CAD build for the part. Positions are in the model's coordinates, mm. A direction names the side the tool comes from. Give positions to 0.01 mm unless a question says otherwise; leave off trailing zeros. Write each loop counter-clockwise with the first axis right and the second up, starting at its lowest first coordinate (ties: lowest second). Pieces come first, ordered by that corner, then holes. Notation, with made-up numbers: (57.5, -25) - (116.5, -25) arc R32 ccw to (116.5, 7) - close; hole circle Ø8 at (74.25, -6). An arc over 180 degrees is marked (long way). Put each result on its own line as item: value. Start each with the question number.
1. Wall check: line 1 (X direction, y = 60, z = 14); line 2 (X direction, y = 100, z = 3); line 3 (Z direction, x = 29, y = 66). Give the ranges that are in metal, low to high.
2. Drop flat-ended pins along their axis: pin 1 (6 mm diameter, centred on y = 28, z = 25.5, fed in from -X); pin 2 (3 mm diameter, centred on x = 20, z = 17, fed in from +Y); pin 3 (12 mm diameter, centred on x = -5, z = 45, fed in from +Y); pin 4 (17 mm diameter, centred on x = 19.5, y = 98, fed in from +Z). Give the stop position or say it passes through.
3. Cut at B-B on y = 60. List the corners of the cut face in (x, z), and give its area (3 significant figures).
4. Tool access for faces 5 (the cylindrical face through (38, 60.8, 2.1)), 6 (the flat face through (-0.6, 15, 27.8)): list every direction of +Z, -Z, +X, -X, +Y, -Y with a clear straight run to the whole face (end or side of a thin tool).
5. Mould opens along X. For faces 1 (the flat face through (31.01, 7.4, 35.92)), 2 (the flat face through (-30.76, 7.4, 36.37)), 3 (the cylindrical face through (10.651, 104.868, 3.944)), 4 (the flat face through (-1, 80, 17)) say: +X half, -X half, draft (parallel to the pull), parting line (faces both ways), or undercut.
6. Cut at A-A on x = 17.5. List the corners of the cut face in (y, z).
7. Cut at D-D on x = -2.5. List the corners of the cut face in (y, z), and give its area (3 significant figures).
8. Cut at C-C on z = 31. List the corners of the cut face in (x, y).
from build123d import *

# Parameters (mm, degrees)
F0_W           = 80
F0_H           = 20
F1_DEPTH       = 120
F0_R           = 12
F2_DEPTH       = 15
F3_W           = 80
F3_H           = 40
F4_DEPTH       = 12
F5_R           = 6
F6_R           = 7
F7_R           = 8
F8_DEPTH       = 20
F10_R          = 20
F11_DEPTH      = 108.7579344444
F11_DEPTH_BACK = 27.4711870131


with BuildPart() as f1:
    # F0 (on Front) → F1 (new body)
    with BuildSketch(Plane.XZ):
        with Locations((0, 10)):
            Rectangle(F0_W, F0_H)
    extrude(amount=-F1_DEPTH)

    # F0 (on Front) → F2 (join)
    with BuildSketch(Plane.XZ):
        with BuildLine():
            Line((40, 20), (21.7702481089, 52.2904962177))
            ThreePointArc((21.7702481089, 52.2904962177), (0, 65), (-21.7702481089, 52.2904962177))
            Line((-21.7702481089, 52.2904962177), (-40, 20))
            Line((-40, 20), (40, 20))
        make_face()
        with Locations((0, 40)):
            Circle(F0_R, mode=Mode.SUBTRACT)
    extrude(amount=-F2_DEPTH)

    # F3 (on face) → F4 (cut)
    with BuildSketch(Plane.XY.offset(20)):
        with Locations((0, 100)):
            Rectangle(F3_W, F3_H)
    extrude(amount=-F4_DEPTH, mode=Mode.SUBTRACT)

    # F5
    f5_edges = [f1.edges().sort_by_distance(p)[0] for p in [
        (0, 80, 8),
    ]]
    fillet(f5_edges, radius=F5_R)

    # F6
    f6_edges = [f1.edges().sort_by_distance(p)[0] for p in [
        (40, 60, 0),
        (-40, 60, 0),
    ]]
    fillet(f6_edges, radius=F6_R)

    # F7 (on face) → F8 (cut, through all)
    with BuildSketch(Plane(origin=(0, 0, 0), x_dir=(1, 0, 0), z_dir=(0, 0, -1))):
        with Locations((17, -60)):
            Circle(F7_R)
        with Locations((17, -100)):
            Circle(F7_R)
        with Locations((-17, -100)):
            Circle(F7_R)
        with Locations((-17, -60)):
            Circle(F7_R)
    extrude(amount=-F8_DEPTH, mode=Mode.SUBTRACT)

    # F10 (on line) → F11 (cut, two sides)
    with BuildSketch(Plane(origin=(0, 0, 0), x_dir=(1, 0, 0), z_dir=(0, -0.906307787, 0.4226182617))) as f11_sk:
        Circle(F10_R)
    extrude(amount=-F11_DEPTH, mode=Mode.SUBTRACT)
    extrude(f11_sk.sketch, amount=F11_DEPTH_BACK, mode=Mode.SUBTRACT)


solid = f1.part
Report:
1. line 1: x = -40 to -25, -9 to 9, 25 to 40
1. line 2: x = -38.74 to -25, -9 to 9, 25 to 38.74
1. line 3: z = 0 to 20
2. pin 1: passes through
2. pin 2: stops at y = 80
2. pin 3: stops at y = 15
2. pin 4: stops at z = 8
3. outline: (-40, 7) arc R7 ccw to (-33, 0) - (-25, 0) - (-25, 20) - (-40, 20) - close; (-9, 0) - (9, 0) - (9, 20) - (-9, 20) - close; (25, 0) - (33, 0) arc R7 ccw to (40, 7) - (40, 20) - (25, 20) - close
3. area: 939 mm²
4. face 5: -Z, +X, +Y, -Y
4. face 6: +Z, +X, -X, +Y
5. face 1: +X half
5. face 2: -X half
5. face 3: undercut
5. face 4: draft
6. outline: (0, 10.68) - (22.91, 0) - (52.02, 0) - (52.02, 20) - (15, 20) - (15, 57.85) - (0, 57.85) - close; (67.98, 0) - (92.02, 0) - (92.02, 8) - (86, 8) arc R6 cw to (80, 14) - (80, 20) - (67.98, 20) - close; (107.98, 0) - (120, 0) - (120, 8) - (107.98, 8) - close
7. outline: (0, 21.89) - (46.95, 0) - (120, 0) - (120, 8) - (86, 8) arc R6 cw to (80, 14) - (80, 20) - (15, 20) - (15, 28.26) - (0, 28.26) - close; (0, 51.74) - (15, 51.74) - (15, 64.87) - (0, 64.87) - close
7. area: 1,730 mm²
8. outline: (-33.79, 0) - (-7.94, 0) - (-7.94, 15) - (-33.79, 15) - close; (7.94, 0) - (33.79, 0) - (33.79, 15) - (7.94, 15) - close
